Autodesk Fusion 360 part; units mm, degrees
sketch "Schizzo1" plane through (0, 0, 0) normal (1, 0, 0) x (0, 1, 0)
  spline S0 degree 4 poles (6.5, 0) (7.1387, -3.4839) (13.3781, -3.3973) (18.2915, -6.9187) (18.8284, -9.0213) knots 0 0 0 0 0 1 1 1 1 1
  line L0 (6.5, 0) -> (7.1387, -3.4839)
  line L1 (7.1387, -3.4839) -> (13.3781, -3.3973)
  line L2 (13.3781, -3.3973) -> (18.2915, -6.9187)
  line L3 (18.2915, -6.9187) -> (18.8284, -9.0213)
  line L4 (3.225, 0) -> (3.225, 15)
  line L5 (15.8979, -3.483) -> (21.2628, -8.3935)
  line L6 (3.225, 0) -> (6.5, 0)
  line L7 (20.25, -9.5) -> (21.75, -9.5) construction
  arc A0 (12.1624, 5) -> (15.8979, -3.483) centre (23.6624, 5) ccw
  line L8 (0, 0) -> (3.225, 0) construction
  line L9 (0, 0) -> (0, 15) construction
  line L10 (3.225, 15) -> (0, 15)
  line L11 (0, 95) -> (0, 15)
  line L12 (20.25, -11) -> (20.25, -9.5) construction
  circle A1 centre (20.25, -9.5) radius 1.5
  line L13 (0, 95) -> (-15, 95) construction
  line L14 (12.1624, 5) -> (12.1624, 50)
  ellipse E0 centre (0, 78.5258) end of major axis (18.2065, 78.5258) minor radius 16.4742 (16.9001, 72.398) -> (0, 95) ccw
  arc A2 (16.9001, 72.398) -> (12.1624, 50) centre (67.476, 50) ccw
  line L15 (0, 81) -> (18, 81) construction
  point P0 (11, 1)
  point P1 (20.25, -11)
  dimension "d1" = 3.225
  dimension "d2" = 15
  dimension "d3" = 6.5
  dimension "d5" = 11
  dimension "d6" = 3
  dimension "d7" = 21.75
  dimension "d8" = 11
  dimension "d9" = 1
  dimension "d17" = 6.24
  dimension "d18" = 3.542
  dimension "d19" = 6.045
  dimension "d20" = 2.17
  dimension "d24" = 11.5
  dimension "d38" = 90
  dimension "d41" = 4
  dimension "d45" = 18
  dimension "d46" = 14
  dimension "d47" = 45
revolve "Rivoluzione1" add sketch "Schizzo1" angle 360 about axis through (0, 0, 95) along (0, 0, -1) contours S0 L1 L2 L3 L4 L5 L6 A0 L10 L11 A1 L14 E0 A2 | A1
chamfer "Smusso1" distance 1 angle 45 1 edges at (-3.0068, 1.1662, 0)
equation "d1 = larghezza_incastro_joystick / 2"
equation "d3 = ( 13 / 2 ) * 1 mm"
equation "d7 = ( 43.5 / 2 ) * 1 mm"
equation "d8 = ( 22 / 2 ) * 1 mm"
equation "altezza_joystick = 90 mm"
equation "larghezza_incastro_joystick = 6.45 mm"
equation "d38 = altezza_joystick"
The listing builds one solid part. Answer for the finished solid, in the listing's coordinates (mm). A direction names the side the tool comes from. Coordinates: 2 decimals unless noted, no trailing zeros. Write each loop counter-clockwise with the first axis right and the second up, starting at its lowest first coordinate (ties: lowest second). Pieces come first, ordered by that corner, then holes. Notation, with made-up numbers: (69.5, 15) - (101.5, 15) arc R20 cw to (101.5, 21) - close; hole circle Ø6 at (82, 7.25). An arc over 180 degrees is marked (long way). Put each result on its own line as item: value.
1. A tool of negligible diameter and unlimited length cuts with its end or side. For faces 4 (the face through (0, 0, 15)), 5 (the face through (11.873, -2.637, 27.815)), from which of +Z, -Z, +X, -X, +Y, -Y can it reach the whole face along a straight path? Write none if from no direction.
Answer sheet:
face 4: -Z
face 5: none
2. Flat-ended cylindrical pins translate along their axes: pin 1 Ø12 at (x, z) = (11.5, 60.5) entering from -Y; pin 2 Ø5 at (x, z) = (-6, 29) entering from -Y; pin 3 Ø5 at (x, y) = (-4.5, 2) entering from +Z. Find the tip coordinate at first contact, or state that the pin passes through.
Answer sheet:
pin 1: stops at y = -12.32
pin 2: stops at y = -11.65
pin 3: stops at z = 94.85
3. The part is cut by section A-A on z = 60.5. Give the vertices of the cut face in (x, y).
Answer sheet:
outline: circle Ø26.34 at (0, 0)
4. Find the intervals of material crossed by line 1 along X through (y, z) = (0, 12) (3 decimals); line 2 along Y through (x, z) = (1.5, 26); line 3 along X through (y, z) = (-3, 83), in increasing order. Write a range as from..to.
Answer sheet:
line 1: x = -12.162..-3.225, 3.225..12.162
line 2: y = -12.07..12.07
line 3: x = -17.26..17.26
5. Determine the mould class of faces 1 (the face through (10.593, -2.352, -3.432)), 2 (the face through (-15.85, -3.52, -3.79)), 3 (the face through (3.15, -0.7, 8.1)) for opening direction Z: pulls with the +Z half, pulls with the -Z half, needs draft (parallel to the pull), parting line crosses it, or undercut.
Answer sheet:
face 1: pulls with the -Z half
face 2: undercut
face 3: needs draft
